Could you check a few things on this model? Use its own coordinates, in mm. Round coordinates to 2 decimals unless told otherwise and drop trailing zeros. Order: outer loops, then holes, each group sorted by start corner. A loop starts at its lowest first (then second) coordinate and runs counter-clockwise, first axis right, second up.
Autodesk Inventor part; units mm, degrees
ref_plane "YZ Plane" through (0, 0, 0) normal (1, 0, 0) x (0, 1, 0)
ref_plane "XZ Plane" through (0, 0, 0) normal (0, 1, 0) x (-1, 0, 0)
ref_plane "XY Plane" through (0, 0, 0) normal (0, 0, 1) x (1, 0, 0)
sketch "Sketch1" plane through (0, 0, 0) normal (0, 0, 1) x (1, 0, 0)
  line L0 (0, 0) -> (-267, 0)
  line L1 (-267, 0) -> (-267, 10)
  line L2 (-267, 10) -> (-263.5, 10)
  line L3 (-263.5, 10) -> (-263.5, 20)
  line L4 (-3.5, 20) -> (-3.5, 10)
  line L5 (-3.5, 10) -> (0, 10)
  line L6 (0, 10) -> (0, 0)
  line L7 (-83.5, 20) -> (-83.5, 25)
  line L8 (-83.5, 25) -> (-183.5, 25)
  line L9 (-183.5, 25) -> (-183.5, 20)
  line L10 (-263.5, 20) -> (-183.5, 20)
  line L11 (-83.5, 20) -> (-3.5, 20)
  dimension "d19" = 267
  dimension "d20" = 10
  dimension "d22" = 10
  dimension "d23" = 260
  dimension "d24" = 100
  dimension "d25" = 5
  dimension "d26" = 80
extrude "Extrusion1" add sketch "Sketch1" along normal blind 3.5
sketch "Sketch2" plane through (0, 0, 3.5) normal (0, 0, 1) x (1, 0, 0)
  line L0 (-267, 0) -> (0, 0) construction
  line L1 (0, 0) -> (0, 10) construction
  line L2 (0, 10) -> (-3.5, 10)
  line L3 (-3.5, 10) -> (-3.5, 20)
  line L4 (-3.5, 20) -> (-83.5, 20) construction
  line L5 (-83.5, 20) -> (-83.5, 25) construction
  line L6 (-83.5, 25) -> (-183.5, 25) construction
  line L7 (-183.5, 25) -> (-183.5, 20) construction
  line L8 (-183.5, 20) -> (-263.5, 20) construction
  line L9 (-263.5, 20) -> (-263.5, 10)
  line L10 (-263.5, 10) -> (-267, 10)
  line L11 (-267, 10) -> (-267, 0) construction
  line L12 (-263.5, 10) -> (-267, 10)
  line L13 (-267, 10) -> (-267, 20)
  line L14 (-267, 20) -> (-263.5, 20)
  line L15 (-263.5, 20) -> (-263.5, 10)
  line L16 (-3.5, 10) -> (0, 10)
  line L17 (0, 10) -> (0, 20)
  line L18 (0, 20) -> (-3.5, 20)
  line L19 (-3.5, 20) -> (-3.5, 10)
extrude "Extrusion2" add sketch "Sketch2" against normal blind 3.5
sketch "Sketch3" plane through (0, 0, 3.5) normal (0, 0, 1) x (1, 0, 0)
  line L0 (-267, 0) -> (0, 0) construction
  line L1 (0, 0) -> (0, 20) construction
  line L2 (0, 20) -> (-83.5, 20) construction
  line L3 (-83.5, 20) -> (-83.5, 25) construction
  line L4 (-83.5, 25) -> (-183.5, 25) construction
  line L5 (-183.5, 25) -> (-183.5, 20) construction
  line L6 (-183.5, 20) -> (-267, 20) construction
  line L7 (-267, 0) -> (-267, 20) construction
  line L8 (-267, 0) -> (-267, 20)
  line L9 (-267, 0) -> (-263.5, 0)
  line L10 (-263.5, 0) -> (-263.5, 10)
  line L11 (-263.5, 10) -> (-267, 10)
  line L12 (-267, 10) -> (-267, 0)
  line L13 (0, 0) -> (-3.5, 0)
  line L14 (-3.5, 0) -> (-3.5, 10)
  line L15 (-3.5, 10) -> (0, 10)
  line L16 (0, 10) -> (0, 0)
  dimension "d29" = 3.5
  dimension "d30" = 10
  dimension "d31" = 3.5
  dimension "d32" = 10
extrude "Extrusion3" cut sketch "Sketch3" against normal blind 3.5
properties part number "Refuerzo_Base"
Q1. For P1, Ø1, axis at x = -215.5, z = 2.5, coming from the +Y side; P2, Ø12, axis at x = -64, y = 5, coming from the -Z side; P3, Ø1.8, axis at y = 23, z = 1.5, coming from the -X side; P4, Ø1.8, axis at x = -265.5, z = 1, coming from the -Y side, each with a flat end and sliding along its axis, tell me the tip position at first contact or that it passes through.
Q2. I need wall thicknesses on L1, parallel to Y at x = -231.5, z = 2.75; L2, parallel to X at y = 20.75, z = 1.8; L3, parallel to X at y = 2.25, z = 3.1. Which ranges of each line are inside material? Lowest first, please.
Q3. Imagine slicing it at A-A, the plane z = 1.6. Please give me the cut outline in (x, y).
Q4. Imagine slicing it at B-B, the plane y = 3.25. Please give me the cut outline in (x, z).
Q5. Imagine slicing it at C-C, the plane x = -192.5. Please give me the cut outline in (y, z).
Filled in:
1. P1: stops at y = 20
1. P2: stops at z = 0
1. P3: stops at x = -183.5
1. P4: stops at y = 10
2. L1: y = 0 to 20
2. L2: x = -183.5 to -83.5
2. L3: x = -263.5 to -3.5
3. outline: (-267, 10) - (-263.5, 10) - (-263.5, 0) - (-3.5, 0) - (-3.5, 10) - (0, 10) - (0, 20) - (-83.5, 20) - (-83.5, 25) - (-183.5, 25) - (-183.5, 20) - (-267, 20) - close
4. outline: (-263.5, 0) - (-3.5, 0) - (-3.5, 3.5) - (-263.5, 3.5) - close
5. outline: (0, 0) - (20, 0) - (20, 3.5) - (0, 3.5) - close
